```python
from build123d import *

# Parameters (mm, degrees)
F0_W     = 101.6
F0_H     = 63.5
F1_DEPTH = 50.8
F2_T     = -2.54
F3_R     = 6.985
F4_DEPTH = 101.601
F5_W     = 50.8
F5_H     = 25.4
F6_DEPTH = 63.501


with BuildPart() as f1:
    # F0 (on Top) → F1 (new body)
    with BuildSketch(Plane.XY):
        Rectangle(F0_W, F0_H)
    extrude(amount=F1_DEPTH)

    # F2
    f2_openings = [f1.faces().sort_by_distance(p)[0] for p in [
        (0, 0, 50.8),
    ]]
    offset(amount=F2_T, openings=f2_openings)

    # F3 (on face) → F4 (cut, through all)
    with BuildSketch(Plane.YZ.offset(50.8)):
        with Locations((0, 25.4)):
            Circle(F3_R)
    extrude(amount=-F4_DEPTH, mode=Mode.SUBTRACT)

    # F5 (on face) → F6 (cut, through all)
    with BuildSketch(Plane.XZ.offset(31.75)):
        with Locations((0, 38.1)):
            Rectangle(F5_W, F5_H)
    extrude(amount=-F6_DEPTH, mode=Mode.SUBTRACT)


solid = f1.part
```
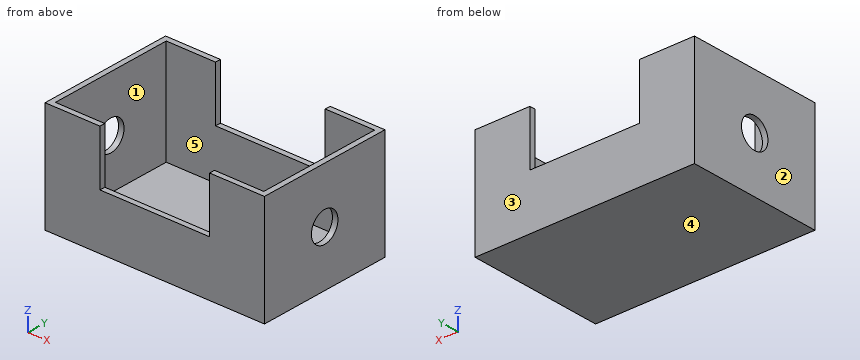
Can you work these out from the model? Positions are in its coordinate system, mm. Face numbers are marked on the shaded views. A direction names the side the tool comes from. Coordinates: 2 decimals unless noted, no trailing zeros. Loops run counter-clockwise (first coordinate to the right, second up) from the corner with the lowest first, then second, coordinate; pieces in that order, holes last. Notation, with made-up numbers: (25, -7.5) -> (45, -7.5) arc R25 ccw to (45, 20.5) -> close; hole circle Ø6 at (6.5, -8.5). An arc over 180 degrees is marked (long way). Put each result on its own line as item: value. Start each with the question number.
Q1. If I drill on line 1 (Y direction, x = -2, z = 25); line 2 (X direction, y = -18, z = 36); line 3 (Y direction, x = -50, z = 25), over which ranges is the centre line in solid material (lowest first)? Write a range as [from, to].
Q2. I want a section at B-B (z = 38). Write out the boundary of the cut face in (x, y), plus the area to 3 significant figures.
Q3. I want a section at C-C (z = 14). Write out the boundary of the cut face in (x, y).
Q4. For the marked faces 4 and 5, which set-ups out of +Z, -Z, +X, -X, +Y, -Y let a thin tool reach every point of the face, with its end or its side?
Q5. I want a section at A-A (y = 0). Write out the boundary of the cut face in (x, z) (3 decimals), plus the area to 3 significant figures.
Q6. I want a section at D-D (x = 1.5). Write out the boundary of the cut face in (y, z).
Q7. Thinking about a two-plate mould opening in X: for the marked faces 1, 2 and 3, which applies, pulls with the +X half, pulls with the -X half, needs draft (parallel to the pull), parting line crosses it, or undercut?
Q8. I'm going to push flat-ended pins straight in: P1, Ø17.5, axis at x = 15.5, y = -14.5, coming from the +Z side; P2, Ø2, axis at x = 9, y = 30.5, coming from the +Z side. Where does each tip first touch, or does it pass through?
Taken from the geometry:
1. line 1: y = [-31.75, -29.21], [29.21, 31.75]
1. line 2: x = [-50.8, -48.26], [48.26, 50.8]
1. line 3: y = [-31.75, -6.97], [6.97, 31.75]
2. outline: (-50.8, -31.75) -> (-25.4, -31.75) -> (-25.4, -29.21) -> (-48.26, -29.21) -> (-48.26, 29.21) -> (-25.4, 29.21) -> (-25.4, 31.75) -> (-50.8, 31.75) -> close; (25.4, -31.75) -> (50.8, -31.75) -> (50.8, 31.75) -> (25.4, 31.75) -> (25.4, 29.21) -> (48.26, 29.21) -> (48.26, -29.21) -> (25.4, -29.21) -> close
2. area: 555 mm2
3. outline: (-50.8, -31.75) -> (50.8, -31.75) -> (50.8, 31.75) -> (-50.8, 31.75) -> close; hole (-48.26, -29.21) -> (48.26, -29.21) -> (48.26, 29.21) -> (-48.26, 29.21) -> close
4. face 4: -Z, +X, -X, +Y, -Y
4. face 5: +Z
5. outline: (-50.8, 0) -> (50.8, 0) -> (50.8, 18.415) -> (48.26, 18.415) -> (48.26, 2.54) -> (-48.26, 2.54) -> (-48.26, 18.415) -> (-50.8, 18.415) -> close; (-50.8, 32.385) -> (-48.26, 32.385) -> (-48.26, 50.8) -> (-50.8, 50.8) -> close; (48.26, 32.385) -> (50.8, 32.385) -> (50.8, 50.8) -> (48.26, 50.8) -> close
5. area: 432 mm2
6. outline: (-31.75, 0) -> (31.75, 0) -> (31.75, 25.4) -> (29.21, 25.4) -> (29.21, 2.54) -> (-29.21, 2.54) -> (-29.21, 25.4) -> (-31.75, 25.4) -> close
7. face 1: undercut
7. face 2: pulls with the -X half
7. face 3: needs draft
8. P1: stops at z = 2.54
8. P2: stops at z = 25.4
